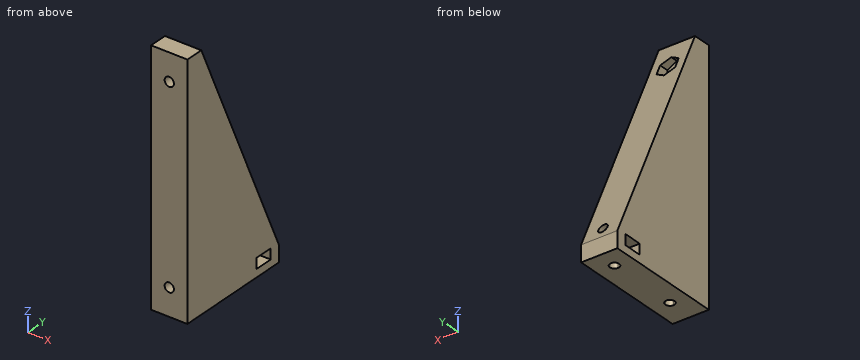
from build123d import *

# Parameters (mm, degrees)
F1_DEPTH  = 20
F3_D      = 5.1
F5_DEPTH  = 12
F6_DEPTH  = 25
F7_DEPTH  = 15
F8_D      = 5.1
F9_W      = 5.1
F9_H      = 5.7
F10_DEPTH = 25
F4_W      = 10
F4_H      = 4
F11_DEPTH = 25


# Not quite as in the source:
# - a feature names something its author has since deleted; it is built from what else it names


with BuildPart() as f1:
    # F0 (on Right) → F1 (new body)
    with BuildSketch(Plane.YZ):
        Polygon((-70, 0), (0, 0), (-60, 135), (-70, 135), align=None)
    extrude(amount=F1_DEPTH)

    # F3 (through all)
    with Locations(Plane.XZ.offset(70)):
        with Locations((10, 15), (10, 120)):
            Hole(F3_D / 2)

    # F4 (on face) → F5 (cut)
    with BuildSketch(Plane(origin=(0, 0, 0), x_dir=(1, 0, 0), z_dir=(0, 0, -1))):
        with BuildLine():
            ThreePointArc((12.55, 55), (11.803122292, 56.803122292), (10, 57.55))
            Line((10, 57.55), (10, 55))
            Line((10, 55), (10, 52.45))
            ThreePointArc((10, 52.45), (11.803122292, 53.196877708), (12.55, 55))
        make_face()
        with BuildLine():
            ThreePointArc((12.55, 15), (11.803122292, 16.803122292), (10, 17.55))
            ThreePointArc((10, 17.55), (8.196877708, 13.196877708), (12.55, 15))
        make_face()
        with BuildLine():
            Line((10, 55), (10, 57.55))
            ThreePointArc((10, 57.55), (7.45, 55), (10, 52.45))
            Line((10, 52.45), (10, 55))
        make_face()
    extrude(amount=-F5_DEPTH, mode=Mode.SUBTRACT)

    # F2 (on face) → F6 (join)
    with BuildSketch(Plane.XZ.offset(70)):
        Polygon((15.1, 122.9444863729), (10, 125.8889727457), (4.9, 122.9444863729), (4.9, 117.0555136271), (10, 114.1110272543), (15.1, 117.0555136271), align=None)
    extrude(amount=-F6_DEPTH)

    # F7 (cut): a face of the model
    f7_faces = [f1.faces().sort_by_distance(p)[0] for p in [
        (10, -45, 120),
    ]]
    extrude(f7_faces, amount=-F7_DEPTH, mode=Mode.SUBTRACT)

    # F8 (through all)
    with Locations(Plane.XZ.offset(70)):
        with Locations((10, 120)):
            Hole(F8_D / 2)

    # F9 (on face) → F10 (cut)
    with BuildSketch(Plane(origin=(0, 0, 0), x_dir=(0, -1, 0), z_dir=(-1, 0, 0))):
        with Locations((12.45, 7.15)):
            Rectangle(F9_W, F9_H)
        with Locations((17.55, 7.15)):
            Rectangle(F9_W, F9_H)
    extrude(amount=-F10_DEPTH, mode=Mode.SUBTRACT)

    # F4 (on face) → F11 (cut)
    with BuildSketch(Plane(origin=(0, 0, 0), x_dir=(1, 0, 0), z_dir=(0, 0, -1))):
        with Locations((15, 2)):
            Rectangle(F4_W, F4_H)
        with Locations((5, 2)):
            Rectangle(F4_W, F4_H)
    extrude(amount=-F11_DEPTH, mode=Mode.SUBTRACT)


solid = f1.part
The model under review builds one solid part; all positions refer to its coordinate system, in mm. Give positions to 0.01 mm unless a question says otherwise; leave off trailing zeros. Write each loop counter-clockwise with the first axis right and the second up, starting at its lowest first coordinate (ties: lowest second). Pieces come first, ordered by that corner, then holes.
1. Add section A-A, the plane y = -39. Write out the cut boundary in (x, z).
2. Add section D-D, the plane z = 45. Write out the cut boundary in (x, y).
3. For P1, Ø2, axis at y = -59.5, z = 61.5, coming from the -X side; P2, Ø11, axis at x = 10.5, z = 119, coming from the +Y side; P3, Ø5, axis at x = 8.5, y = -16.5, coming from the +Z side; P4, Ø10, axis at x = 10.5, z = 43, coming from the +Y side, all flat-tipped, find the tip position at first contact; note any pin that passes through.
4. Add section B-B, the plane x = 1.5. Write out the cut boundary in (y, z).
5. Wall thickness on L1, parallel to Z at x = 10, y = -64; L2, parallel to Y at x = 10, z = 3.4; L3, parallel to Y at x = 10, z = 10.55: over which ranges is each line inside the solid? List them lowest first.
6. Add section C-C, the plane z = 120. Write out the cut boundary in (x, y).
Worked answers:
1. outline: (0, 0) - (20, 0) - (20, 87.75) - (0, 87.75) - close; hole circle Ø5.1 at (10, 15)
2. outline: (0, -70) - (20, -70) - (20, -20) - (0, -20) - close
3. P1: stops at x = 0
3. P2: stops at y = -50.44
3. P3: stops at z = 42.75
3. P4: stops at y = -16.89
4. outline: (-70, 0) - (-4, 0) - (-4, 9) - (-60, 135) - (-70, 135) - close; hole (-20.1, 4.3) - (-9.9, 4.3) - (-9.9, 10) - (-20.1, 10) - close
5. L1: z = 0 to 12.45, 17.55 to 117.45, 122.55 to 135
5. L2: y = -70 to -57.55, -52.45 to -17.55, -12.45 to -4
5. L3: y = -70 to -57.55, -52.45 to -17.55, -12.45 to -4.69
6. outline: (0, -70) - (7.45, -70) - (7.45, -60) - (4.9, -60) - (4.9, -53.33) - (0, -53.33) - close; (12.55, -70) - (20, -70) - (20, -53.33) - (15.1, -53.33) - (15.1, -60) - (12.55, -60) - close
